Autodesk Inventor part; units mm, degrees
ref_plane "YZ Plane" through (0, 0, 0) normal (1, 0, 0) x (0, 1, 0)
ref_plane "XZ Plane" through (0, 0, 0) normal (0, 1, 0) x (-1, 0, 0)
ref_plane "XY Plane" through (0, 0, 0) normal (0, 0, 1) x (1, 0, 0)
sketch "Sketch1" plane through (0, 0, 0) normal (0, 0, 1) x (1, 0, 0)
  circle A0 centre (0, 0) radius 9.9
  dimension "d0" = 19.8
extrude "Extrusion1" add sketch "Sketch1" along normal blind 2
sketch "Sketch2" plane through (0, 0, 2) normal (0, 0, 1) x (1, 0, 0)
  circle A0 centre (0, 0) radius 8.9
  dimension "d3" = 17.8
extrude "Extrusion2" add sketch "Sketch2" along normal blind 4
thread "Thread1"
sketch "Sketch3" plane through (0, 0, 0) normal (0, 0, -1) x (-1, 0, 0)
  circle A0 centre (0, 0) radius 4
  dimension "d8" = 8
extrude "Extrusion3" cut sketch "Sketch3" against normal blind 10
properties part number "punta"
Geometry: final body of the model. Coordinates: model frame, mm. A direction names the side the tool comes from. Round coordinates to 2 decimals unless told otherwise and drop trailing zeros. Order: outer loops, then holes, each group sorted by start corner. A loop starts at its lowest first (then second) coordinate and runs counter-clockwise, first axis right, second up. Notation, with made-up numbers: (42.5, 30.5) - (80.5, 30.5) arc R5 cw to (80.5, 38.5) - close; hole circle Ø2 at (70, 42). An arc over 180 degrees is marked (long way). Write item = value, one per line. Start each with the question number.
Q1. Pull-direction query (X, two-part tool) for faces 1 (the cylindrical face through (-1.93, 8.69, 3.97)), 2 (the cylindrical face through (0.867, -3.905, 2.958)), 3 (the flat face through (-0.1, -4.3, 0)); classes: +X half, -X half, draft (parallel to the pull), parting line (faces both ways), or undercut.
Q2. Cut plane D-D on y = 6.75. Return the cut outline in (x, z).
Q3. Ray query, line 1 (Y direction, x = 0, z = 4.3); line 2 (Z direction, x = -1, y = -9); line 3 (X direction, y = -0.75, z = 5.75). Return the intervals inside material, ascending. Write a range as from..to.
Q4. Access query for faces 4 (the cylindrical face through (9.443, -2.974, 0.986)), 5 (the flat face through (-9, 2, 2)). Directions: +Z, -Z, +X, -X, +Y, -Y. A direction counts if a zero-diameter tool reaches every point of the face in a straight line with its end or side. Return the directions, or none.
Q5. Cut plane C-C on z = 1.3. Return the cut outline in (x, y), and give its area (3 significant figures).
Q6. Pin query (flat end, axial travel): pin 1 (2 mm diameter, centred on y = 7, z = 4, fed in from +X); pin 2 (1.5 mm diameter, centred on y = -4.5, z = 2, fed in from +X); pin 3 (2 mm diameter, centred on x = 4, z = 0.5, fed in from +Y). Return the tip coordinate at first contact, or that it passes through.
Q7. Cut plane A-A on x = 0. Return the cut outline in (y, z).
Outcome:
q1.face_1 = parting line
q1.face_2 = undercut
q1.face_3 = draft
q2.outline = (-7.24, 0) - (7.24, 0) - (7.24, 2) - (5.8, 2) - (5.8, 6) - (-5.8, 6) - (-5.8, 2) - (-7.24, 2) - close
q3.line_1 = -8.9..-4, 4..8.9
q3.line_2 = 0..2
q3.line_3 = -8.87..-3.93, 3.93..8.87
q4.face_4 = +Z, -Z
q4.face_5 = +Z
q5.outline = circle Ø19.8 at (0, 0); hole circle Ø8 at (0, 0)
q5.area = 258 mm^2
q6.pin_1 = 6.57
q6.pin_2 = 9.16
q6.pin_3 = 9.43
q7.outline = (-9.9, 0) - (-4, 0) - (-4, 6) - (-8.9, 6) - (-8.9, 2) - (-9.9, 2) - close; (4, 0) - (9.9, 0) - (9.9, 2) - (8.9, 2) - (8.9, 6) - (4, 6) - close
